Geometry check sheet. Reference: the model listing, model coordinates, mm. Face numbers are marked on the shaded views. A direction names the side the tool comes from. Give positions to 0.01 mm unless a question says otherwise; leave off trailing zeros. Loops run counter-clockwise (first coordinate to the right, second up) from the corner with the lowest first, then second, coordinate; pieces in that order, holes last.
1. Tool access check on the marked faces 4 and 5. Record the directions out of +Z, -Z, +X, -X, +Y, -Y that give a thin tool (end or side, any length) a straight path to the whole face; none if there is none.
2. Go/stop test with flat-tipped pins: pin 1 Ø3.5 at (x, y) = (7.07, 0) entering from -Z; pin 2 Ø1.5 at (x, z) = (8, -2) entering from +Y; pin 3 Ø3.5 at (y, z) = (9.5, 0) entering from +X; pin 4 Ø1.7 at (y, z) = (-9.5, 0) entering from -X. Record where each tip stops, or that it passes through.
3. Cross-section at C-C, the plane y = 0. Record the cut outline in (x, z).
4. Material ranges on L1, parallel to Y at x = 3.1, z = 0; L2, parallel to Z at x = 4.25, y = 4.5; L3, parallel to X at y = -1.25, z = -5.25, recorded low to high.
5. Cross-section at B-B, the plane x = 4.5. Record the cut outline in (y, z).
6. Release check for a two-part mould opening along Y. For the marked faces 1, 2 and 3 record: +Y half, -Y half, draft (parallel to the pull), parting line (faces both ways), or undercut.
7. Cross-section at A-A, the plane z = 0. Record the cut outline in (x, y).
8. Cross-section at D-D, the plane y = 9.5. Record the cut outline in (x, z).
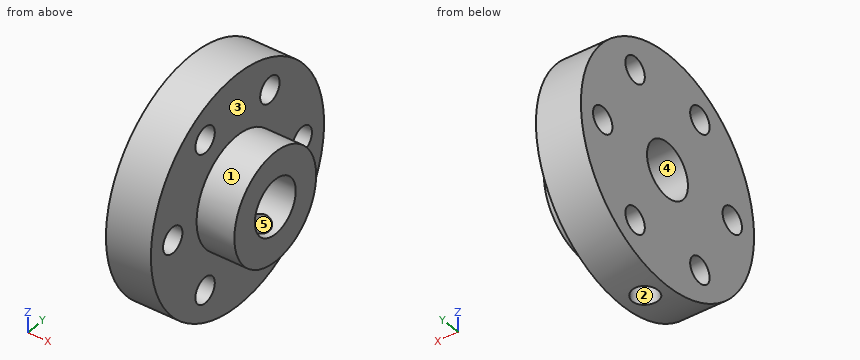
from build123d import *

# Parameters (mm, degrees)
SKETCH1_R           = 12.7
BOSS_EXTRUDE1_DEPTH = 9.2
CUT_EXTRUDE1_START  = -4.2
SKETCH2_R           = 12.7
SKETCH2_R_2         = 6
CUT_EXTRUDE1_DEPTH  = 4.2
SKETCH4_R           = 3
SKETCH4_R_2         = 1.4224
CUT_EXTRUDE2_DEPTH  = 21.179692763
SKETCH5_R           = 1.4224
CUT_EXTRUDE3_DEPTH  = 21.179692763


with BuildPart() as part:
    # Sketch1 → Boss-Extrude1 (new body)
    with BuildSketch(Plane(origin=(0, 0, 0), x_dir=(0, 0, -1), z_dir=(1, 0, 0))):
        Circle(SKETCH1_R)
    extrude(amount=BOSS_EXTRUDE1_DEPTH)

    # Sketch2 → Cut-Extrude1 (cut)
    with BuildSketch(Plane(origin=(9.2, 0, 0), x_dir=(0, 0, -1), z_dir=(1, 0, 0)).offset(CUT_EXTRUDE1_START)):
        Circle(SKETCH2_R)
        Circle(SKETCH2_R_2, mode=Mode.SUBTRACT)
    extrude(amount=CUT_EXTRUDE1_DEPTH, mode=Mode.SUBTRACT)

    # Sketch4 → Cut-Extrude2 (cut, through all)
    with BuildSketch(Plane.ZY):
        Circle(SKETCH4_R)
        with Locations((-8.227241336, -4.75)):
            Circle(SKETCH4_R_2)
        with Locations((8.227241336, 4.75)):
            Circle(SKETCH4_R_2)
        with Locations((-8.227241336, 4.75)):
            Circle(SKETCH4_R_2)
        with Locations((0, 9.5)):
            Circle(SKETCH4_R_2)
        with Locations((0, -9.5)):
            Circle(SKETCH4_R_2)
        with Locations((8.227241336, -4.75)):
            Circle(SKETCH4_R_2)
    extrude(amount=-CUT_EXTRUDE2_DEPTH, mode=Mode.SUBTRACT)

    # Sketch5 → Cut-Extrude3 (cut, through all)
    with BuildSketch(Plane.XY):
        with Locations((2.469287496, 0)):
            Circle(SKETCH5_R)
        with Locations((7.069287496, 0)):
            Circle(SKETCH5_R)
    extrude(amount=-CUT_EXTRUDE3_DEPTH, mode=Mode.SUBTRACT)


solid = part.part
Result:
1. face 4: +X, -X
1. face 5: -Z
2. pin 1: stops at z = -6
2. pin 2: stops at y = 5.87
2. pin 3: stops at x = 5
2. pin 4: passes through
3. outline: (0, -12.7) - (1.05, -12.7) - (1.05, -3) - (0, -3) - close; (0, 3) - (9.2, 3) - (9.2, 6) - (5, 6) - (5, 12.7) - (0, 12.7) - close; (3.89, -12.7) - (5, -12.7) - (5, -6) - (5.65, -6) - (5.65, -3) - (3.89, -3) - close; (8.49, -6) - (9.2, -6) - (9.2, -3) - (8.49, -3) - close
4. L1: y = -12.7 to -10.92, -8.08 to -3, 3 to 8.08, 10.92 to 12.7
4. L2: z = -11.88 to -9.63, -6.83 to 6.83, 9.63 to 11.88
4. L3: x = 0 to 1.79, 3.15 to 6.39, 7.75 to 9.2
5. outline: circle Ø25.4 at (0, 0); hole circle Ø2.84 at (-9.5, 0); hole circle Ø2.84 at (-4.75, -8.23); hole circle Ø2.84 at (-4.75, 8.23); hole circle Ø6 at (0, 0); hole circle Ø2.84 at (4.75, -8.23); hole circle Ø2.84 at (4.75, 8.23); hole circle Ø2.84 at (9.5, 0)
6. face 1: parting line
6. face 2: undercut
6. face 3: draft
7. outline: (0, -12.7) - (5, -12.7) - (5, -10.92) - (0, -10.92) - close; (0, -8.08) - (5, -8.08) - (5, -6) - (9.2, -6) - (9.2, -3) - (0, -3) - close; (0, 3) - (9.2, 3) - (9.2, 6) - (5, 6) - (5, 8.08) - (0, 8.08) - close; (0, 10.92) - (5, 10.92) - (5, 12.7) - (0, 12.7) - close
8. outline: (0, -8.43) - (5, -8.43) - (5, -1.42) - (0, -1.42) - close; (0, 1.42) - (5, 1.42) - (5, 8.43) - (0, 8.43) - close
